Work out the finished part from the listing and answer in its coordinate system (mm). A direction names the side the tool comes from. Round coordinates to 2 decimals unless told otherwise and drop trailing zeros. Order: outer loops, then holes, each group sorted by start corner. A loop starts at its lowest first (then second) coordinate and runs counter-clockwise, first axis right, second up. Notation, with made-up numbers: (66.5, -17.5) - (103.5, -17.5) arc R29 cw to (103.5, 2.5) - close; hole circle Ø3 at (14, 10.25). An arc over 180 degrees is marked (long way). Use one line per item in the form item = value. Start each with the question number.
Q1. Given P1, Ø3.5, axis at x = 150.76, y = 0, coming from the +Z side; P2, Ø1, axis at x = 150, y = -10.5, coming from the +Z side; P3, Ø6, axis at x = 144.5, z = 2.5, coming from the -Y side; P4, Ø8, axis at y = -25.5, z = 9, coming from the +X side, each flat-ended and moving along its own axis, determine where each tip first touches the part or whether it passes through.
Q2. The part is cut by section A-A on y = 0. Determine the outline of the cut face in (x, z), plus the area to 3 significant figures.
Q3. The part is cut by section B-B on z = 9.75. Determine the outline of the cut face in (x, y).
Q4. The part is cut by section D-D on y = -26.5. Determine the outline of the cut face in (x, z).
Q5. The part is cut by section C-C on z = 14.25. Determine the outline of the cut face in (x, y), plus the area to 3 significant figures.
Q6. Find the intervals of material crossed by line 1 (Z direction, x = 152.5, y = 19.5); line 2 (Y direction, x = 150.75, z = 1); line 3 (X direction, y = 28, z = 1), in increasing order. Write a range as [from, to].
Q7. For a pull along Y with two mould halves and no side action, classify faces 1 (the flat face through (156, 0, 17)), 2 (the cylindrical face through (148.762, 0.088, 5.423)), 3 (the cylindrical face through (145, -0.5, 5.4)), 4 (the flat face through (145.536, -38.996, 6.492)) as +Y half, -Y half, draft (parallel to the pull), parting line (faces both ways), or undercut.
Q8. Which of the six approach directions +Z, -Z, +X, -X, +Y, -Y give full straight-line access (tool end or side, diameter ignored) to faces 5 (the flat face through (148, 1, 0)), 6 (the cylindrical face through (155, -0.6, 14))?
from build123d import *

# Parameters (mm, degrees)
F0_R     = 156.5
F0_R_2   = 155
F2_DEPTH = 17
F1_R     = 156.5
F1_R_2   = 2
F1_R_3   = 145
F3_DEPTH = 11
F5_DEPTH = 25


with BuildPart() as f2:
    # F0 (on Top) → F2 (new body)
    with BuildSketch(Plane.XY):
        Circle(F0_R)
        Circle(F0_R_2, mode=Mode.SUBTRACT)
    extrude(amount=F2_DEPTH)

    # F1 (on face) → F3 (join)
    with BuildSketch(Plane.XY):
        Circle(F1_R)
        with Locations((-75.380214, -130.56236)):
            Circle(F1_R_2, mode=Mode.SUBTRACT)
        with Locations((-130.56236, -75.380214)):
            Circle(F1_R_2, mode=Mode.SUBTRACT)
        with Locations((0, -150.760427)):
            Circle(F1_R_2, mode=Mode.SUBTRACT)
        with Locations((75.380214, -130.56236)):
            Circle(F1_R_2, mode=Mode.SUBTRACT)
        with Locations((130.56236, -75.380214)):
            Circle(F1_R_2, mode=Mode.SUBTRACT)
        with Locations((-150.760427, 0)):
            Circle(F1_R_2, mode=Mode.SUBTRACT)
        with Locations((-130.56236, 75.380214)):
            Circle(F1_R_2, mode=Mode.SUBTRACT)
        with Locations((-75.380214, 130.56236)):
            Circle(F1_R_2, mode=Mode.SUBTRACT)
        Circle(F1_R_3, mode=Mode.SUBTRACT)
        with Locations((150.760427, 0)):
            Circle(F1_R_2, mode=Mode.SUBTRACT)
        with Locations((130.56236, 75.380214)):
            Circle(F1_R_2, mode=Mode.SUBTRACT)
        with Locations((0, 150.760427)):
            Circle(F1_R_2, mode=Mode.SUBTRACT)
        with Locations((75.380214, 130.56236)):
            Circle(F1_R_2, mode=Mode.SUBTRACT)
    extrude(amount=F3_DEPTH)

    # F4 (on Top) → F5 (intersect)
    with BuildSketch(Plane.XY):
        Polygon((186.290355, 49.91635), (0, 0), (186.290355, -49.91635), align=None)
    extrude(amount=F5_DEPTH, mode=Mode.INTERSECT)


solid = f2.part
Found:
q1.P1 = through
q1.P2 = 11
q1.P3 = -39.52
q1.P4 = 155.02
q2.outline = (145, 0) - (148.76, 0) - (148.76, 11) - (145, 11) - close; (152.76, 0) - (156.5, 0) - (156.5, 17) - (155, 17) - (155, 11) - (152.76, 11) - close
q2.area = 91.5 mm²
q3.outline = (140.06, -37.53) - (151.17, -40.51) arc R156.5 ccw to (151.17, 40.51) - (140.06, 37.53) arc R145 cw to start; hole circle Ø4 at (150.76, 0)
q4.outline = (142.56, 0) - (154.24, 0) - (154.24, 17) - (152.72, 17) - (152.72, 11) - (142.56, 11) - close
q5.outline = (149.72, -40.12) - (151.17, -40.51) arc R156.5 ccw to (151.17, 40.51) - (149.72, 40.12) arc R155 cw to start
q5.area = 122 mm²
q6.line_1 = [0, 11]
q6.line_2 = [-40.39, -2], [2, 40.39]
q6.line_3 = [142.27, 153.97]
q7.face_1 = draft
q7.face_2 = undercut
q7.face_3 = undercut
q7.face_4 = -Y half
q8.face_5 = -Z, +X, -X, +Y, -Y
q8.face_6 = +Z, -X
